```python
from build123d import *

# Parameters (mm, degrees)
SKETCH1_W           = 211
SKETCH1_H           = 390
SKETCH1_W_2         = 99
SKETCH1_H_2         = 150
SKETCH1_W_3         = 66
SKETCH1_H_3         = 152
BOSS_EXTRUDE1_DEPTH = 3
SKETCH2_R           = 2.6
CUT_EXTRUDE1_DEPTH  = 348.276906805


with BuildPart() as part:
    # Sketch1 → Boss-Extrude1 (new body)
    with BuildSketch(Plane.XY):
        with Locations((51, -115)):
            Rectangle(SKETCH1_W, SKETCH1_H)
        Rectangle(SKETCH1_W_2, SKETCH1_H_2, mode=Mode.SUBTRACT)
        with Locations((102, 0)):
            Rectangle(SKETCH1_W_2, SKETCH1_H_2, mode=Mode.SUBTRACT)
        with Locations((48.5, -229)):
            Rectangle(SKETCH1_W_3, SKETCH1_H_3, mode=Mode.SUBTRACT)
    extrude(amount=BOSS_EXTRUDE1_DEPTH)

    # Sketch2 → Cut-Extrude1 (cut, through all)
    with BuildSketch(Plane.XY.offset(3)):
        with Locations((-24, -134)):
            Circle(SKETCH2_R)
        with Locations((126, -134)):
            Circle(SKETCH2_R)
        with Locations((126, -284)):
            Circle(SKETCH2_R)
        with Locations((-24, -284)):
            Circle(SKETCH2_R)
    extrude(amount=-CUT_EXTRUDE1_DEPTH, mode=Mode.SUBTRACT)


solid = part.part
```
The listing builds one solid part. Answer for the finished solid, in the listing's coordinates (mm). Give positions to 0.01 mm unless a question says otherwise; leave off trailing zeros. Write each loop counter-clockwise with the first axis right and the second up, starting at its lowest first coordinate (ties: lowest second). Pieces come first, ordered by that corner, then holes. Notation, with made-up numbers: (78, 56) -> (127, 56) arc R22 cw to (127, 65) -> close; hole circle Ø1 at (29.25, 30). An arc over 180 degrees is marked (long way). Use one line per item in the form item = value.
1) Section D-D on z = 1.5 is taken. Write down the section's boundary in (x, y).
Result:
outline = (-54.5, -310) -> (156.5, -310) -> (156.5, 80) -> (-54.5, 80) -> close; hole (-49.5, -75) -> (49.5, -75) -> (49.5, 75) -> (-49.5, 75) -> close; hole circle Ø5.2 at (-24, -284); hole circle Ø5.2 at (-24, -134); hole (15.5, -305) -> (81.5, -305) -> (81.5, -153) -> (15.5, -153) -> close; hole (52.5, -75) -> (151.5, -75) -> (151.5, 75) -> (52.5, 75) -> close; hole circle Ø5.2 at (126, -284); hole circle Ø5.2 at (126, -134)
2) Section A-A on y = -262 is taken. Write down the section's boundary in (x, z).
Result:
outline = (-54.5, 0) -> (15.5, 0) -> (15.5, 3) -> (-54.5, 3) -> close; (81.5, 0) -> (156.5, 0) -> (156.5, 3) -> (81.5, 3) -> close
3) Section C-C on y = 43.5 is taken. Write down the section's boundary in (x, z).
Result:
outline = (-54.5, 0) -> (-49.5, 0) -> (-49.5, 3) -> (-54.5, 3) -> close; (49.5, 0) -> (52.5, 0) -> (52.5, 3) -> (49.5, 3) -> close; (151.5, 0) -> (156.5, 0) -> (156.5, 3) -> (151.5, 3) -> close
4) Section B-B on x = -33 is taken. Write down the section's boundary in (y, z).
Result:
outline = (-310, 0) -> (-75, 0) -> (-75, 3) -> (-310, 3) -> close; (75, 0) -> (80, 0) -> (80, 3) -> (75, 3) -> close
5) Straight lines are drawn through the part: probe 1 along X at (y, z) = (-13.5, 2.7); probe 2 along X at (y, z) = (-284, 1.35); probe 3 along Y at (x, z) = (58.5, 2.3). For each, find the intervals that lie inside material, in ascending order.
Result:
probe_1 = -54.5 to -49.5, 49.5 to 52.5, 151.5 to 156.5
probe_2 = -54.5 to -26.6, -21.4 to 15.5, 81.5 to 123.4, 128.6 to 156.5
probe_3 = -310 to -305, -153 to -75, 75 to 80
